from build123d import *

# Parameters (mm, degrees)
SKETCH1_R           = 2.65
BOSS_EXTRUDE1_DEPTH = 20
SKETCH2_W           = 20.3
SKETCH2_H           = 10
SKETCH2_R           = 2.65
SKETCH2_W_2         = 2.5
SKETCH2_H_2         = 5.6
BOSS_EXTRUDE2_DEPTH = 7
SKETCH3_R           = 1.65
CUT_EXTRUDE5_DEPTH  = 10
FILLET1_R           = 1
SKETCH7_W           = 3.85
SKETCH7_H           = 5.298601426
SKETCH7_W_2         = 5.298601426
SKETCH7_H_2         = 3.85
CUT_EXTRUDE6_DEPTH  = 20


with BuildPart() as part:
    # Sketch1 → Boss-Extrude1 (new body)
    with BuildSketch(Plane.XY):
        with BuildLine():
            Line((4.092676386, 16.5), (2.649300713, 14))
            Line((2.649300713, 14), (-2.649300713, 14))
            Line((-2.649300713, 14), (-4.092676386, 16.5))
            ThreePointArc((-4.092676386, 16.5), (-12.02081528, 12.02081528), (-16.5, 4.092676386))
            Line((-16.5, 4.092676386), (-14, 2.649300713))
            Line((-14, 2.649300713), (-14, -2.649300713))
            Line((-14, -2.649300713), (-16.5, -4.092676386))
            ThreePointArc((-16.5, -4.092676386), (-12.02081528, -12.02081528), (-4.092676386, -16.5))
            Line((-4.092676386, -16.5), (-2.649300713, -14))
            Line((-2.649300713, -14), (2.649300713, -14))
            Line((2.649300713, -14), (4.092676386, -16.5))
            ThreePointArc((4.092676386, -16.5), (12.02081528, -12.02081528), (16.5, -4.092676386))
            Line((16.5, -4.092676386), (14, -2.649300713))
            Line((14, -2.649300713), (14, 2.649300713))
            Line((14, 2.649300713), (16.5, 4.092676386))
            ThreePointArc((16.5, 4.092676386), (12.02081528, 12.02081528), (4.092676386, 16.5))
        make_face()
        Circle(SKETCH1_R, mode=Mode.SUBTRACT)
    extrude(amount=BOSS_EXTRUDE1_DEPTH)

    # Sketch2 → Boss-Extrude2 (add)
    with BuildSketch(Plane.XY.offset(20)):
        Rectangle(SKETCH2_W, SKETCH2_H)
        Circle(SKETCH2_R, mode=Mode.SUBTRACT)
        with Locations((-5.9, 0)):
            Rectangle(SKETCH2_W_2, SKETCH2_H_2, mode=Mode.SUBTRACT)
        with Locations((5.9, 0)):
            Rectangle(SKETCH2_W_2, SKETCH2_H_2, mode=Mode.SUBTRACT)
    extrude(amount=BOSS_EXTRUDE2_DEPTH)

    # Sketch3 → Cut-Extrude5 (cut)
    with BuildSketch(Plane.ZY.offset(10.15)):
        with Locations((23.5, 0)):
            Circle(SKETCH3_R)
    extrude(amount=-CUT_EXTRUDE5_DEPTH, mode=Mode.SUBTRACT)

    # Fillet1
    fillet1_edges = [part.edges().sort_by_distance(p)[0] for p in [
        (10.15, 0, 27),
        (0, 5, 27),
        (-10.15, 0, 27),
        (0, -5, 27),
        (10.15, -5, 23.5),
        (10.15, 5, 23.5),
        (-10.15, 5, 23.5),
        (-10.15, -5, 23.5),
    ]]
    fillet(fillet1_edges, radius=FILLET1_R)

    # Cut-Sweep2: sweep along a path in Sketch6
    with BuildLine(Plane.XY.offset(20)) as cut_sweep2_path:
        CenterArc((0, 0), 17, 0, 360)
    # Sketch5 → Cut-Sweep2 (sweep, cut)
    with BuildSketch(Plane(origin=(-4.075202292, 2.35281914, 0), x_dir=(0, 0, 1), z_dir=(-0.8660254037844398, 0.499999999999998, 0))):
        Polygon((9, 13.449006009), (11, 13.449006009), (16, 16.335757355), (4, 16.335757355), align=None)
    sweep(path=cut_sweep2_path.line, mode=Mode.SUBTRACT)

    # Sketch7 → Cut-Extrude6 (cut)
    with BuildSketch(Plane.XY.offset(20)):
        with Locations((-12.075, 0)):
            Rectangle(SKETCH7_W, SKETCH7_H)
        with Locations((0, 12.075)):
            Rectangle(SKETCH7_W_2, SKETCH7_H_2)
        with Locations((12.075, 0)):
            Rectangle(SKETCH7_W, SKETCH7_H)
        with Locations((0, -12.075)):
            Rectangle(SKETCH7_W_2, SKETCH7_H_2)
    extrude(amount=-CUT_EXTRUDE6_DEPTH, mode=Mode.SUBTRACT)


solid = part.part
Verification items for the finished model (mm, model axes). A direction names the side the tool comes from. Coordinates: 2 decimals unless noted, no trailing zeros. Order: outer loops, then holes, each group sorted by start corner. A loop starts at its lowest first (then second) coordinate and runs counter-clockwise, first axis right, second up. Notation, with made-up numbers: M 36,7.5 L 50,7.5 A19 ccw 50,30.5 Z; hole C -19,4.25 d9. An arc over 180 degrees is marked long. Return JSON: item names as keys, results as strings.
1) Gauge pin test, flat ends, axial feed: pin 1 (10 mm diameter, centred on x = 11.5, z = 12.5, fed in from -Y); pin 2 (6 mm diameter, centred on x = -1, z = 7, fed in from -Y); pin 3 (3 mm diameter, centred on y = -1, z = 23.5, fed in from +X). Record the tip position at first contact, or that the pin passes through.
Answer list:
{"pin 1": "y = -15.04", "pin 2": "y = -15.71", "pin 3": "x = 10.15"}
2) Access from +Z, -Z, +X, -X, +Y, -Y to the whole of each face (thin tool, end or side, straight path). Record for faces 5 (the flat face through (6, 0, 20)), 6 (the flat face through (-14.95, -3.2, 3.44)), 7 (the cylindrical face through (-9.865, -4.699, 23.042)), 8 (the flat face through (14.95, 3.2, 16.44)), 9 (the flat face through (0, 10.15, 10)).
Answer list:
{"face 5": "+Z", "face 6": "+Z, -Z, -X", "face 7": "+Z, -X, -Y", "face 8": "+Z, -Z, +X", "face 9": "+Z, -Z, +Y"}
3) Cross-section at D-D, the plane x = 14.5. Count the separate pieces of the cut face and the enclosed holes in it, and give its area (3 significant figures).
Answer list:
{"separate pieces": "4", "enclosed holes": "0", "area": "149 mm2"}
4) Cross-section at B-B, the plane x = 0. Record the boundary of the cut face in (y, z), and give its area (3 significant figures).
Answer list:
{"outline": "M -10.15,0 L -2.65,0 L -2.65,27 L -4,27 A1 ccw -5,26 L -5,20 L -10.15,20 Z; M 2.65,0 L 10.15,0 L 10.15,20 L 5,20 L 5,26 A1 ccw 4,27 L 2.65,27 Z", "area": "332 mm2"}
5) Cross-section at A-A, the plane y = 0. Record the boundary of the cut face in (x, z).
Answer list:
{"outline": "M -10.15,0 L -2.65,0 L -2.65,21.85 L -4.65,21.85 L -4.65,20 L -7.15,20 L -7.15,21.85 L -10.15,21.85 Z; M -10.15,25.15 L -7.15,25.15 L -7.15,27 L -9.15,27 A1 ccw -10.15,26 Z; M -4.65,25.15 L -2.65,25.15 L -2.65,27 L -4.65,27 Z; M 2.65,0 L 10.15,0 L 10.15,26 A1 ccw 9.15,27 L 7.15,27 L 7.15,20 L 4.65,20 L 4.65,27 L 2.65,27 Z"}
6) Release check for a two-part mould opening along X. For faces 1 (the cylindrical face through (-11.93, 12.11, 17.97)), 2 (the flat face through (3.2, -14.95, 16.44)), 3 (the flat face through (-3.2, 14.95, 16.44)), 4 (the flat face through (-2, 2, 27)) record: +X half, -X half, draft (parallel to the pull), parting line (faces both ways), or undercut.
Answer list:
{"face 1": "-X half", "face 2": "undercut", "face 3": "undercut", "face 4": "draft"}
7) Thickness scan on L1, parallel to Y at x = 13, z = 6; L2, parallel to X at y = 0, z = 12.75; L3, parallel to Y at x = -3.45, z = 23.5. Record the ranges inside material, lowest first. Write a range as [from, to].
Answer list:
{"L1": "[-9.14, -2.65], [2.65, 9.14]", "L2": "[-10.15, -2.65], [2.65, 10.15]", "L3": "[-5, -1.65], [1.65, 5]"}
8) Cross-section at C-C, the plane z = 23.5. Record the boundary of the cut face in (x, y).
Answer list:
{"outline": "M -10.15,-4 A1 ccw -9.15,-5 L 9.15,-5 A1 ccw 10.15,-4 L 10.15,4 A1 ccw 9.15,5 L -9.15,5 A1 ccw -10.15,4 L -10.15,1.65 L -7.15,1.65 L -7.15,2.8 L -4.65,2.8 L -4.65,1.65 L -2.07,1.65 A2.65 cw long -2.07,-1.65 L -4.65,-1.65 L -4.65,-2.8 L -7.15,-2.8 L -7.15,-1.65 L -10.15,-1.65 Z; hole M 4.65,-2.8 L 7.15,-2.8 L 7.15,2.8 L 4.65,2.8 Z"}
